Build history of the part. All positions in model axes, mm. Round coordinates to 2 decimals unless told otherwise and drop trailing zeros. Loops run counter-clockwise (first coordinate to the right, second up) from the corner with the lowest first, then second, coordinate; pieces in that order, holes last. Notation, with made-up numbers: (88.5, -7.5) - (113.5, -7.5) arc R30 ccw to (113.5, 18.5) - close; hole circle Ø11 at (80, 9). An arc over 180 degrees is marked (long way). Use a Markdown table: item, result.
Autodesk Fusion 360 part; units mm, degrees
sketch "Sketch1" plane through (0, 0, 0) normal (0, 0, 1) x (1, 0, 0)
  line L0 (0, 40.6706) -> (170.6716, 40.6706)
  line L1 (170.6716, 40.6706) -> (170.6716, 0)
  line L2 (170.6716, 0) -> (0, 0)
  line L3 (0, 0) -> (0, 40.6706)
sketch "Sketch2" plane through (0, 0, 0) normal (0, 0, 1) x (1, 0, 0)
  circle A0 centre (2.5, 4) radius 1.75
  line L0 (170.6716, 0) -> (0, 0)
  line L1 (0, 0) -> (0, 40.6706)
  dimension "d1" = 3.5
  dimension "d2" = 4
  dimension "d3" = 2.5
sketch "Sketch4" plane through (0, 0, 0) normal (0, 0, 1) x (1, 0, 0)
  circle A0 centre (49.5, 4) radius 1.75
  circle A1 centre (2.5, 4) radius 1.75
  dimension "d9" = 3.5
  dimension "d10" = 47
extrude "Extrude1" add sketch "Sketch1" along normal blind 4
sketch "Sketch11" plane through (0, 0, 4) normal (0, 0, 1) x (-1, 0, 0)
  line L0 (0, 0) -> (-170.6716, 0)
  line L1 (-170.6716, 0) -> (-170.6716, -40.6706)
  line L2 (-170.6716, -40.6706) -> (0, -40.6706)
  line L3 (0, -40.6706) -> (0, 0)
  line L4 (-5, -30) -> (-150, -30)
  line L5 (-150, -30) -> (-150, -10)
  line L6 (-150, -10) -> (-5, -10)
  line L7 (-5, -10) -> (-5, -30)
sketch "Sketch13" plane through (0, 0, 4) normal (0, 0, 1) x (-1, 0, 0)
  line L0 (0, 0) -> (-170.6716, 0)
  line L1 (-170.6716, 0) -> (-170.6716, -40.6706)
  line L2 (-170.6716, -40.6706) -> (0, -40.6706)
  line L3 (0, -40.6706) -> (0, 0)
  circle A0 centre (-8, -4) radius 1.75
  circle A1 centre (-8, -36) radius 1.75
  circle A2 centre (-50.5, -36) radius 1.75
  circle A3 centre (-50.5, -4) radius 1.75
  circle A4 centre (-120.5, -4) radius 1.75
  circle A5 centre (-120.5, -36) radius 1.75
  circle A6 centre (-166.5, -4) radius 1.75
  circle A7 centre (-166.5, -36) radius 1.75
  dimension "d44" = 3.5
  dimension "d45" = 4
  dimension "d46" = 3.5
  dimension "d47" = 32
  dimension "d48" = 8
  dimension "d49" = 8
  dimension "d50" = 3.5
  dimension "d52" = 3.5
  dimension "d53" = 4
  dimension "d55" = 32
  dimension "d56" = 3.5
  dimension "d58" = 4
  dimension "d59" = 3.5
  dimension "d60" = 32
  dimension "d62" = 3.5
  dimension "d63" = 46
  dimension "d64" = 4
  dimension "d65" = 3.5
  dimension "d66" = 46
  dimension "d67" = 32
extrude "Extrude5" cut sketch "Sketch13" against normal blind 15 contours A0 | A1 | A2 | A3 | A4 | A5 | A6 | A7
sketch "Sketch16" plane through (0, 0, 4) normal (0, 0, 1) x (-1, 0, 0)
  circle A0 centre (-120.5, -36) radius 1.75
  circle A1 centre (-50.5, -36) radius 1.75
  circle A2 centre (-50.5, -4) radius 1.75
  circle A3 centre (-120.5, -4) radius 1.75
  circle A4 centre (-166.5, -36) radius 1.75
  circle A5 centre (-8, -36) radius 1.75
  circle A6 centre (-8, -4) radius 1.75
  circle A7 centre (-166.5, -4) radius 1.75
  line L0 (0, 0) -> (-170.6716, 0)
  line L1 (-170.6716, 0) -> (-170.6716, -40.6706)
  line L2 (-170.6716, -40.6706) -> (0, -40.6706)
  line L3 (0, -40.6706) -> (0, 0)
  line L4 (-5, -33) -> (-27, -33)
  line L5 (-27, -33) -> (-27, -31)
  line L6 (-27, -31) -> (-5, -31)
  line L7 (-5, -31) -> (-5, -33)
  line L8 (-5, -6.9037) -> (-25, -6.9037)
  line L9 (-25, -6.9037) -> (-25, -8.99)
  line L10 (-25, -8.99) -> (-5, -8.99)
  line L11 (-5, -8.99) -> (-5, -6.9037)
  line L12 (-5, -28.024) -> (-10, -28.024)
  line L13 (-10, -28.024) -> (-10, -12)
  line L14 (-10, -12) -> (-5, -12)
  line L15 (-5, -12) -> (-5, -28.024)
  line L16 (-15, -28) -> (-20, -28)
  line L17 (-20, -28) -> (-20, -12)
  line L18 (-20, -12) -> (-15, -12)
  line L19 (-15, -12) -> (-15, -28)
  line L20 (-25.2942, -28) -> (-30, -28)
  line L21 (-30, -28) -> (-30, -12)
  line L22 (-30, -12) -> (-25.2942, -12)
  line L23 (-25.2942, -12) -> (-25.2942, -28)
  line L24 (-30, -33) -> (-43, -33)
  line L25 (-43, -33) -> (-43, -31)
  line L26 (-43, -31) -> (-30, -31)
  line L27 (-30, -31) -> (-30, -33)
  line L28 (-30, -9) -> (-43, -9)
  line L29 (-43, -9) -> (-43, -7)
  line L30 (-43, -7) -> (-30, -7)
  line L31 (-30, -7) -> (-30, -9)
  circle A8 centre (-55, -20) radius 14.1421
  line L32 (-94.9908, -12) -> (-100.1485, -12)
  line L33 (-100.1485, -12) -> (-100.1485, -30)
  line L34 (-100.1485, -30) -> (-94.9908, -30)
  line L35 (-94.9908, -30) -> (-94.9908, -12)
  line L36 (-114.4734, -27.5201) -> (-119.9683, -27.5201)
  line L37 (-119.9683, -27.5201) -> (-119.9683, -11.6326)
  line L38 (-119.9683, -11.6326) -> (-114.4734, -11.6326)
  line L39 (-114.4734, -11.6326) -> (-114.4734, -27.5201)
  line L40 (-134.7975, -27.5201) -> (-140.4499, -27.5201)
  line L41 (-140.4499, -27.5201) -> (-140.4499, -12)
  line L42 (-140.4499, -12) -> (-134.7975, -12)
  line L43 (-134.7975, -12) -> (-134.7975, -27.5201)
  line L44 (-154.7885, -27.5201) -> (-160.2653, -27.5201)
  line L45 (-160.2653, -27.5201) -> (-160.2653, -12)
  line L46 (-160.2653, -12) -> (-154.7885, -12)
  line L47 (-154.7885, -12) -> (-154.7885, -27.5201)
  line L48 (-75, -10) -> (-100, -10)
  line L49 (-100, -10) -> (-100, -7.452)
  line L50 (-100, -7.452) -> (-75, -7.452)
  line L51 (-75, -7.452) -> (-75, -10)
  line L52 (-110, -8.9897) -> (-139.8992, -8.9897)
  line L53 (-139.8992, -8.9897) -> (-139.8992, -6.7652)
  line L54 (-139.8992, -6.7652) -> (-110, -6.7652)
  line L55 (-110, -6.7652) -> (-110, -8.9897)
  line L56 (-145, -9.7245) -> (-165.0971, -9.7245)
  line L57 (-165.0971, -9.7245) -> (-165.0971, -7.5785)
  line L58 (-165.0971, -7.5785) -> (-145, -7.5785)
  line L59 (-145, -7.5785) -> (-145, -9.7245)
  line L60 (-75, -35) -> (-99.8075, -35)
  line L61 (-99.8075, -35) -> (-99.8075, -32.5523)
  line L62 (-99.8075, -32.5523) -> (-75, -32.5523)
  line L63 (-75, -32.5523) -> (-75, -35)
  line L64 (-110, -32.4558) -> (-136, -32.4558)
  line L65 (-136, -32.4558) -> (-136, -29.8985)
  line L66 (-136, -29.8985) -> (-110, -29.8985)
  line L67 (-110, -29.8985) -> (-110, -32.4558)
  line L68 (-145, -31.9897) -> (-167, -31.9897)
  line L69 (-167, -31.9897) -> (-167, -29.9185)
  line L70 (-167, -29.9185) -> (-145, -29.9185)
  line L71 (-145, -29.9185) -> (-145, -31.9897)
  dimension "d78" = 22
  dimension "d79" = 3
  dimension "d81" = 13
  dimension "d82" = 13
extrude "Extrude8" cut sketch "Sketch16" against normal blind 15 contours L4 L5 L6 L7 | L8 L9 L10 L11 | L12 L13 L14 L15 | L16 L17 L18 L19 | L20 L21 L22 L23 | L24 L25 L26 L27 | L28 L29 L30 L31 | A8 | L32 L33 L34 L35 | L36 L37 L38 L39 | L40 L41 L42 L43 | L44 L45 L46 L47 | L48 L49 L50 L51 | L52 L53 L54 L55 | L56 L57 L58 L59 | L60 L61 L62 L63 | L64 L65 L66 L67 | L68 L69 L70 L71
Q1. Cut at B-B, the plane y = 4. List the corners of the cut face in (x, z).
Results found:
| item | result |
|---|---|
| outline | (0, 0) - (6.25, 0) - (6.25, 4) - (0, 4) - close; (9.75, 0) - (48.75, 0) - (48.75, 4) - (9.75, 4) - close; (52.25, 0) - (118.75, 0) - (118.75, 4) - (52.25, 4) - close; (122.25, 0) - (164.75, 0) - (164.75, 4) - (122.25, 4) - close; (168.25, 0) - (170.67, 0) - (170.67, 4) - (168.25, 4) - close |
Q2. Cut at A-A, the plane x = 8. List the corners of the cut face in (y, z).
Results found:
| item | result |
|---|---|
| outline | (0, 0) - (2.25, 0) - (2.25, 4) - (0, 4) - close; (5.75, 0) - (6.9, 0) - (6.9, 4) - (5.75, 4) - close; (8.99, 0) - (12, 0) - (12, 4) - (8.99, 4) - close; (28.02, 0) - (31, 0) - (31, 4) - (28.02, 4) - close; (33, 0) - (34.25, 0) - (34.25, 4) - (33, 4) - close; (37.75, 0) - (40.67, 0) - (40.67, 4) - (37.75, 4) - close |
Q3. Cut at C-C, the plane x = 113. List the corners of the cut face in (y, z), plus the area to 3 significant figures.
Results found:
| item | result |
|---|---|
| outline | (0, 0) - (6.77, 0) - (6.77, 4) - (0, 4) - close; (8.99, 0) - (29.9, 0) - (29.9, 4) - (8.99, 4) - close; (32.46, 0) - (40.67, 0) - (40.67, 4) - (32.46, 4) - close |
| area | 144 mm2 |
Q4. Probe line 1 (X direction, y = 4, z = 2.15); line 2 (Y direction, x = 89, z = 1.4); line 3 (Y direction, x = 147, z = 1.5). List the from-to ranges inside material, lowest first.
Results found:
| item | result |
|---|---|
| line 1 | x = 0 to 6.25, 9.75 to 48.75, 52.25 to 118.75, 122.25 to 164.75, 168.25 to 170.67 |
| line 2 | y = 0 to 7.45, 10 to 32.55, 35 to 40.67 |
| line 3 | y = 0 to 7.58, 9.72 to 29.92, 31.99 to 40.67 |
Q5. Pull direction X, two halves, no side cores. Call faces 1 (the face through (123, 29.898, 2)), 2 (the face through (87, 0, 2)): pulls with the +X half, pulls with the -X half, needs draft (parallel to the pull), parting line crosses it, or undercut.
Results found:
| item | result |
|---|---|
| face 1 | undercut |
| face 2 | needs draft |
Q6. Cut at D-D, the plane x = 50.5. List the corners of the cut face in (y, z), plus the area to 3 significant figures.
Results found:
| item | result |
|---|---|
| outline | (0, 0) - (2.25, 0) - (2.25, 4) - (0, 4) - close; (5.75, 0) - (6.59, 0) - (6.59, 4) - (5.75, 4) - close; (33.41, 0) - (34.25, 0) - (34.25, 4) - (33.41, 4) - close; (37.75, 0) - (40.67, 0) - (40.67, 4) - (37.75, 4) - close |
| area | 27.4 mm2 |
